from build123d import *

# Parameters (mm, degrees)
BOSS_EXTRUDE1_DEPTH = 2.54
FILLET1_R           = 6.35


with BuildPart() as part:
    # Sketch1 → Boss-Extrude1 (new body)
    with BuildSketch(Plane(origin=(0, 0, 0), x_dir=(1, 0, 0), z_dir=(0, 1, 0))):
        Polygon((-9.525, 12.7), (-22.225, 25.4), (-50.8, 25.4), (-50.8, 5.08), (-53.34, 5.08), (-53.34, -5.08), (-50.8, -5.08), (-50.8, -25.4), (-22.225, -25.4), (-9.525, -12.7), (9.525, -12.7), (22.225, -25.4), (50.8, -25.4), (50.8, -5.08), (53.34, -5.08), (53.34, 5.08), (50.8, 5.08), (50.8, 25.4), (22.225, 25.4), (9.525, 12.7), align=None)
    extrude(amount=BOSS_EXTRUDE1_DEPTH)

    # Fillet1
    fillet1_edges = [part.edges().sort_by_distance(p)[0] for p in [
        (50.8, 1.27, -25.4),
        (50.8, 1.27, 25.4),
        (-50.8, 1.27, 25.4),
        (-50.8, 1.27, -25.4),
    ]]
    fillet(fillet1_edges, radius=FILLET1_R)


solid = part.part
Verification items for the finished model (mm, model axes). A direction names the side the tool comes from. Coordinates: 2 decimals unless noted, no trailing zeros. Order: outer loops, then holes, each group sorted by start corner. A loop starts at its lowest first (then second) coordinate and runs counter-clockwise, first axis right, second up. Notation, with made-up numbers: (31, 19) -> (47, 19) arc R23 ccw to (47, 42) -> close; hole circle Ø1 at (-24.75, 33). An arc over 180 degrees is marked (long way). Put each result on its own line as item: value. Start each with the question number.
1. Cross-section at B-B, the plane z = 20. Record the boundary of the cut face in (x, y) (3 decimals).
2. Cross-section at C-C, the plane x = -1.5. Record the boundary of the cut face in (y, z), then the cut area to 3 significant figures.
3. Mould release check, pull along X, two halves, no side actions. Record for faces 1 (the cylindrical face through (48.89, 1.29, 23.59)), 2 (the flat face through (15.786, 1.252, 18.961)), 3 (the flat face through (33, 1, 25.4)): released by +X, released by -X, zero draft, split by the parting line, or undercut.
4. Access from +Z, -Z, +X, -X, +Y, -Y to the whole of each face (thin tool, end or side, straight path). Record for faces 4 (the flat face through (0, 1, 12.7)), 5 (the flat face through (50.8, 1, -12)), 6 (the flat face through (-52, 1, 5.08)), 7 (the flat face through (50.8, 1, 12)), 8 (the flat face through (15.964, 1.252, -19.139)).
5. Material ranges on L1, parallel to X at y = 0.55, z = -8; L2, parallel to X at y = 1.1, z = 17 (3 decimals); L3, parallel to X at y = 2.4, z = 15 (3 decimals), recorded low to high. Write a range as [from, to].
6. Cross-section at A-A, the plane y = 1.15. Record the boundary of the cut face in (x, z) (3 decimals).
7. Go/stop test with flat-tipped pins: pin 1 Ø1.3 at (y, z) = (1.5, 12) entering from +X; pin 2 Ø4 at (x, z) = (-39.5, 9.5) entering from -Y; pin 3 Ø0.8 at (x, y) = (52, 1.5) entering from -Z; pin 4 Ø1.3 at (x, y) = (3.5, 0.5) entering from -Z. Record where each tip stops, or that it passes through.
8. Cross-section at D-D, the plane z = -16. Record the boundary of the cut face in (x, y) (3 decimals).
Computed:
1. outline: (-50.729, 0) -> (-16.825, 0) -> (-16.825, 2.54) -> (-50.729, 2.54) -> close; (16.825, 0) -> (50.729, 0) -> (50.729, 2.54) -> (16.825, 2.54) -> close
2. outline: (0, -12.7) -> (2.54, -12.7) -> (2.54, 12.7) -> (0, 12.7) -> close
2. area: 64.5 mm2
3. face 1: released by +X
3. face 2: undercut
3. face 3: zero draft
4. face 4: +Z, +Y, -Y
4. face 5: -Z, +X, +Y, -Y
4. face 6: +Z, -X, +Y, -Y
4. face 7: +Z, +X, +Y, -Y
4. face 8: -Z, +Y, -Y
5. L1: [-50.8, 50.8]
5. L2: [-50.8, -13.825], [13.825, 50.8]
5. L3: [-50.8, -11.825], [11.825, 50.8]
6. outline: (-53.34, -5.08) -> (-50.8, -5.08) -> (-50.8, -19.05) arc R6.35 ccw to (-44.45, -25.4) -> (-22.225, -25.4) -> (-9.525, -12.7) -> (9.525, -12.7) -> (22.225, -25.4) -> (44.45, -25.4) arc R6.35 ccw to (50.8, -19.05) -> (50.8, -5.08) -> (53.34, -5.08) -> (53.34, 5.08) -> (50.8, 5.08) -> (50.8, 19.05) arc R6.35 ccw to (44.45, 25.4) -> (22.225, 25.4) -> (9.525, 12.7) -> (-9.525, 12.7) -> (-22.225, 25.4) -> (-44.45, 25.4) arc R6.35 ccw to (-50.8, 19.05) -> (-50.8, 5.08) -> (-53.34, 5.08) -> close
7. pin 1: x = 50.8
7. pin 2: y = 0
7. pin 3: z = -5.08
7. pin 4: z = -12.7
8. outline: (-50.8, 0) -> (-12.825, 0) -> (-12.825, 2.54) -> (-50.8, 2.54) -> close; (12.825, 0) -> (50.8, 0) -> (50.8, 2.54) -> (12.825, 2.54) -> close
